Part model, mm, in its own coordinate system. Face numbers are marked on the shaded views. Round coordinates to 2 decimals unless told otherwise and drop trailing zeros. Loops run counter-clockwise (first coordinate to the right, second up) from the corner with the lowest first, then second, coordinate; pieces in that order, holes last.
(1) Mould opens along X. For the marked faces 1, 2 and 3 say: +X half, -X half, draft (parallel to the pull), parting line (faces both ways), or undercut.
(2) Cut at B-B on x = 11.25. List the corners of the cut face in (y, z) (3 decimals), then the cut area to 3 significant figures.
(3) Cut at A-A on z = -11.5. List the corners of the cut face in (x, y) (3 decimals).
(4) Cut at D-D on y = 13. List the corners of the cut face in (x, z) (3 decimals).
(5) Probe probe 1 along Z at (x, y) = (6.75, 36.5) (3 decimals); probe 2 along X at (y, z) = (86, -8.5) (3 decimals); probe 3 along X at (y, z) = (147.32, -0.75) (1 decimal). List the from-to ranges inside material, lowest first.
(6) Flat gauge pin, fed straight in: pin 1 (4 mm diameter, centred on x = 9, z = -5.5, fed in from -Y). Where does the tip first touch, or does it go through?
Autodesk Inventor part; units mm, degrees
ref_plane "YZ Plane" through (0, 0, 0) normal (1, 0, 0) x (0, 1, 0)
ref_plane "XZ Plane" through (0, 0, 0) normal (0, 1, 0) x (-1, 0, 0)
ref_plane "XY Plane" through (0, 0, 0) normal (0, 0, 1) x (1, 0, 0)
sketch "Sketch1" plane through (0, 0, 0) normal (0, 1, 0) x (-1, 0, 0)
  line L0 (0, 0) -> (-15.875, 0)
  line L1 (-15.875, 0) -> (-15.875, -15.875)
  line L2 (-15.875, -15.875) -> (0, -15.875)
  line L3 (0, -15.875) -> (0, 0)
  dimension "d0" = 15.875
  dimension "d1" = 15.875
extrude "Extrusion1" add sketch "Sketch1" along normal blind 152.4
sketch "Sketch2" plane through (0, 0, 0) normal (0, -1, 0) x (1, 0, 0)
  line L0 (15.875, 0) -> (15.875, -15.875)
  line L1 (0, 0) -> (15.875, 0)
  line L2 (0, -15.875) -> (0, 0)
  line L3 (15.875, -15.875) -> (0, -15.875)
  line L4 (14.2748, -14.2748) -> (14.2748, -1.6002)
  line L5 (14.2748, -1.6002) -> (1.6002, -1.6002)
  line L6 (1.6002, -1.6002) -> (1.6002, -14.2748)
  line L7 (1.6002, -14.2748) -> (14.2748, -14.2748)
  dimension "d4" = 1.6002
extrude "Extrusion2" cut sketch "Sketch2" against normal blind 152.4 contours L7 L6 L5 L4
fillet "Fillet1" radius 1.524 4 edges at (14.2748, 76.2, -14.2748) (1.6002, 76.2, -1.6002) (14.2748, 76.2, -1.6002) (1.6002, 76.2, -14.2748)
fillet "Fillet2" radius 0.254 4 edges at (15.875, 76.2, 0) (15.875, 76.2, -15.875) (0, 76.2, -15.875) (0, 76.2, 0)
sketch "Sketch3" plane through (0.254, 0, 0) normal (0, 0, 1) x (1, 0, 0)
  line L0 (15.367, 152.4) -> (0, 152.4)
  line L1 (7.6835, 152.4) -> (7.6835, 147.32)
  circle A0 centre (7.6835, 147.32) radius 1.905
  point P0 (-0.254, 0)
  dimension "d9" = 5.08
  dimension "d10" = 3.81
extrude "Extrusion3" cut sketch "Sketch3" against normal blind 15.875
sketch "Sketch4" plane through (0.254, 0, 0) normal (0, 0, 1) x (1, 0, 0)
  circle A0 centre (7.6835, 147.32) radius 1.905
  line L0 (7.6835, 147.32) -> (7.6835, 117.221)
  circle A1 centre (7.6835, 115.316) radius 1.905
  point P0 (-0.254, 0)
  dimension "d13" = 30.099
extrude "Extrusion4" cut sketch "Sketch4" against normal blind 15.875 contours A1
properties part number "am-3594 5-8x5-8 0.063 wall tubing"
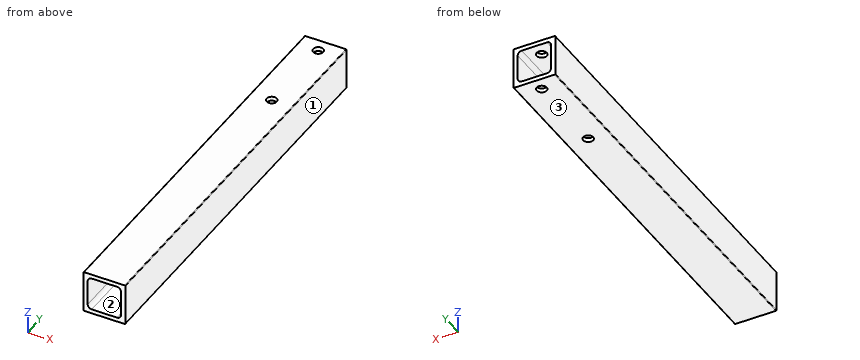
Final values:
1. face 1: +X half
1. face 2: undercut
1. face 3: draft
2. outline: (0, -15.875) - (152.4, -15.875) - (152.4, -14.275) - (0, -14.275) - close; (0, -1.6) - (152.4, -1.6) - (152.4, 0) - (0, 0) - close
2. area: 488 mm2
3. outline: (0, 0) - (1.6, 0) - (1.6, 152.4) - (0, 152.4) - close; (14.275, 0) - (15.875, 0) - (15.875, 152.4) - (14.275, 152.4) - close
4. outline: (0, -15.621) arc R0.254 ccw to (0.254, -15.875) - (15.621, -15.875) arc R0.254 ccw to (15.875, -15.621) - (15.875, -0.254) arc R0.254 ccw to (15.621, 0) - (0.254, 0) arc R0.254 ccw to (0, -0.254) - close; hole (1.6, -12.751) arc R1.524 ccw to (3.124, -14.275) - (12.751, -14.275) arc R1.524 ccw to (14.275, -12.751) - (14.275, -3.124) arc R1.524 ccw to (12.751, -1.6) - (3.124, -1.6) arc R1.524 ccw to (1.6, -3.124) - close
5. probe 1: z = -15.875 to -14.275, -1.6 to 0
5. probe 2: x = 0 to 1.6, 14.275 to 15.875
5. probe 3: x = 0 to 6, 9.8 to 15.9
6. pin 1: passes through
